Autodesk Inventor part; units mm, degrees
ref_plane "Work Plane1" through (0, 0, 3.81) normal (0, 0, 1) x (1, 0, 0)
ref_plane "YZ Plane" through (0, 0, 0) normal (1, 0, 0) x (0, 1, 0)
ref_plane "XZ Plane" through (0, 0, 0) normal (0, 1, 0) x (-1, 0, 0)
sketch "Sketch3" plane through (0, 0, 0) normal (0, 0, 1) x (1, 0, 0)
  circle A0 centre (0, 0) radius 5.08
  dimension "d0" = 10.16
extrude "Extrusion1" add sketch "Sketch3" along normal blind 2.54
ref_plane "Work Plane1" through (0, 0, 3.81) normal (0, 0, 1) x (1, 0, 0)
sketch "Sketch4" plane through (0, 0, 3.81) normal (0, 0, 1) x (1, 0, 0)
  circle A0 centre (0, 0) radius 3.7389
  dimension "d4" = 7.4778
loft "Loft1" add profiles "Sketch4" section 2 edges at (-5.08, 0, 2.54)
sketch "Sketch5" plane through (0, 0, 3.81) normal (0, 0, 1) x (1, 0, 0)
  line L0 (-1.5443, -1.5992) -> (-0.7742, -1.5992)
  line L1 (-0.7742, -1.5992) -> (-0.7742, 1.5992)
  line L2 (-0.7742, 1.5992) -> (-1.5443, 1.5992)
  line L3 (-1.5443, 1.5992) -> (-1.5443, -1.5992)
  line L4 (0.7742, -1.5992) -> (1.5443, -1.5992)
  line L5 (1.5443, -1.5992) -> (1.5443, 1.5992)
  line L6 (1.5443, 1.5992) -> (0.7742, 1.5992)
  line L7 (0.7742, 1.5992) -> (0.7742, -1.5992)
  point P0 (0, 0)
  dimension "d9" = 0.7742
  dimension "d10" = 0.7742
  dimension "d11" = 1.5443
  dimension "d12" = 1.5443
  dimension "d23" = 1.5992
  dimension "d24" = 1.5992
extrude "Extrusion2" add sketch "Sketch5" along normal blind 0.5161
sketch "Sketch6" plane through (-1.5443, -1.5992, 3.81) normal (0, -1, 0) x (1, 0, 0)
  circle A0 centre (0.384, 0.2581) radius 0.1676
  circle A1 centre (2.7046, 0.2581) radius 0.1676
  line L0 (0.7701, 0) -> (0.7701, 0.5161)
  line L1 (2.3185, 0) -> (2.3185, 0.5161)
  line L2 (-2.1946, 0) -> (5.2832, 0)
  point P0 (1.5443, -3.81)
  dimension "d15" = 0.3353
  dimension "d16" = 0.3353
  dimension "d17" = 0.3861
  dimension "d18" = 0.3861
  dimension "d25" = 0.2581
  dimension "d26" = 0.2581
  dimension "d27" = 0.5161
extrude "Extrusion3" cut sketch "Sketch6" against normal blind 2.54
equation "\"d4\" = 0.736 * d0"
equation "\"d13\" = 0.0508 * d0"
equation "\"d15\" = 0.033 * d0"
equation "\"d16\" = d15"
equation "\"d17\" = 0.038 * d0"
equation "\"d18\" = d17"
equation "\"d25\" = 0.5 * d27"
equation "\"d26\" = d25"
properties part number "Dynamic Driver"
Source: CAD feature listing. Evaluate the final solid. Frame: model axes, mm. Coordinates: 2 decimals unless noted, no trailing zeros. Loops run counter-clockwise (first coordinate to the right, second up) from the corner with the lowest first, then second, coordinate; pieces in that order, holes last. Notation, with made-up numbers: M 89.5,27.5 L 130.5,27.5 A19 ccw 130.5,33.5 Z; hole C 67.25,38 d10. An arc over 180 degrees is marked long. Answer in a Markdown table with one row per item.
Q1. Section C-C on y = -0.5. State how many separate pieces and enclosed holes the cut face has, plus the area to 3 significant figures.
Answers below:
| item | result |
|---|---|
| separate pieces | 1 |
| enclosed holes | 2 |
| area | 37.4 mm^2 |
Q2. First-contact query: pin 1 (6 mm diameter, centred on x = -2.5, y = 2.5, fed in from +Z); pin 2 (0.6 mm diameter, centred on y = 0, z = 4, fed in from +X); pin 3 (3 mm diameter, centred on x = -3.5, y = -3.5, fed in from +Z); pin 4 (0.6 mm diameter, centred on y = -0.5, z = 4, fed in from +X). Flat tips, straight axial feed; report the tip coordinate or a pass-through.
Answers below:
| item | result |
|---|---|
| pin 1 | stops at z = 4.33 |
| pin 2 | stops at x = 3.86 |
| pin 3 | stops at z = 3.81 |
| pin 4 | stops at x = 3.82 |
Q3. Section D-D on z = 3.25. Return the cut outline in (x, y).
Answers below:
| item | result |
|---|---|
| outline | C 0,0 d8.66 |
Q4. Section A-A on x = 0. Return the cut outline in (y, z), plus the area to 3 significant figures.
Answers below:
| item | result |
|---|---|
| outline | M -5.08,0 L 5.08,0 L 5.08,2.54 L 3.74,3.81 L -3.74,3.81 L -5.08,2.54 Z |
| area | 37.0 mm^2 |
Q5. Section B-B on z = 1.2. Return the cut outline in (x, y), plus the area to 3 significant figures.
Answers below:
| item | result |
|---|---|
| outline | C 0,0 d10.16 |
| area | 81.1 mm^2 |
Q6. Ray query, probe 1 along Z at (x, y) = (-2.25, 1.75); probe 2 along X at (y, z) = (-1.75, 0.55); probe 3 along X at (y, z) = (-4.25, 2.7). Return the intervals inside material, ascending. Write a range as from..to.
Answers below:
| item | result |
|---|---|
| probe 1 | z = 0..3.81 |
| probe 2 | x = -4.77..4.77 |
| probe 3 | x = -2.46..2.46 |
